Geometry check sheet. Reference: the model listing, model coordinates, mm. A direction names the side the tool comes from. Round coordinates to 2 decimals unless told otherwise and drop trailing zeros. Order: outer loops, then holes, each group sorted by start corner. A loop starts at its lowest first (then second) coordinate and runs counter-clockwise, first axis right, second up. Notation, with made-up numbers: (41, 32) - (80, 32) arc R20 cw to (80, 55) - close; hole circle Ø8 at (54, -21.5). An arc over 180 degrees is marked (long way). One line per question, with ' | ' between items. Start each with the question number.
Q1. Material ranges on line 1 along Y through (x, z) = (5, 25); line 2 along X through (y, z) = (15.5, 14.5); line 3 along Y through (x, z) = (38.1, 48.1), recorded low to high.
Q2. Tool access check on faces 1 (the face through (86.21, 34.72, 2.21)), 2 (the face through (107.95, 38, 26)), 3 (the face through (76.39, 41.44, 5.34)), 4 (the face through (13.99, 59.256, 47.669)), 5 (the face through (48, 0, 46)). Record the directions out of +Z, -Z, +X, -X, +Y, -Y that give a thin tool (end or side, any length) a straight path to the whole face; none if there is none.
Q3. Sectioned sample at D-D, the plane z = 12. Enter the section's corners in (x, y).
Q4. Sectioned sample at A-A, the plane y = 53. Enter the section's corners in (x, z).
Q5. Sectioned sample at C-C, the plane z = 25.4. Enter the section's corners in (x, y), then the cut area to 3 significant figures.
Q6. Sectioned sample at B-B, the plane x = 67. Enter the section's corners in (y, z), then the cut area to 3 significant figures.
Q7. Mould release check, pull along X, two halves, no side actions. Record for faces 6 (the face through (48, 76.2, 46)), 7 (the face through (0, 38, 26)), 8 (the face through (114.3, 38, 26)), 9 (the face through (109.934, 20.9, 21.6)): +X half, -X half, draft (parallel to the pull), parting line (faces both ways), or undercut.
```python
from build123d import *

# Parameters (mm, degrees)
SKETCH1_W           = 114.3
SKETCH1_H           = 50.8
SKETCH1_W_2         = 101.6
SKETCH1_H_2         = 38.1
BOSS_EXTRUDE1_DEPTH = 76.2
CUT_EXTRUDE1_REACH  = 148.464
SKETCH2_R           = 2.4765
SKETCH2_5_R         = 3.81
CUT_EXTRUDE2_DEPTH  = 147.463544952
SKETCH5_R           = 3.81
CUT_EXTRUDE4_DEPTH  = 147.463544952
SKETCH6_R           = 3.81
CUT_EXTRUDE5_DEPTH  = 147.463544952
SKETCH7_R           = 8.73125
CUT_EXTRUDE6_DEPTH  = 1.984375
SKETCH8_R           = 8.73125
CUT_EXTRUDE7_DEPTH  = 1.984375
CUT_EXTRUDE8_START  = -1.984375
SKETCH9_R           = 8.73125
CUT_EXTRUDE8_DEPTH  = 1.984375
CUT_EXTRUDE9_START  = -1.984375
SKETCH10_R          = 8.73125
CUT_EXTRUDE9_DEPTH  = 1.984375


with BuildPart() as part:
    # Sketch1 → Boss-Extrude1 (new body)
    with BuildSketch(Plane(origin=(0, 0, 0), x_dir=(1, 0, 0), z_dir=(0, 1, 0))):
        with Locations((57.15, -25.4)):
            Rectangle(SKETCH1_W, SKETCH1_H)
        with Locations((57.15, -25.4)):
            Rectangle(SKETCH1_W_2, SKETCH1_H_2, mode=Mode.SUBTRACT)
    extrude(amount=BOSS_EXTRUDE1_DEPTH)

    # Sketch2 → Cut-Extrude1 (cut, up to next)
    with BuildSketch(Plane.XY.offset(50.8), mode=Mode.PRIVATE) as cut_extrude1_sk1:
        with Locations((14.526827682, 61.673172318)):
            Circle(SKETCH2_R)
    cut_extrude1_tool1 = extrude(cut_extrude1_sk1.sketch, amount=-CUT_EXTRUDE1_REACH, mode=Mode.PRIVATE) & part.part
    # Sketch2 → Cut-Extrude1 (cut, up to next)
    with BuildSketch(Plane.XY.offset(50.8), mode=Mode.PRIVATE) as cut_extrude1_sk2:
        with Locations((61.673172318, 61.673172318)):
            Circle(SKETCH2_R)
    cut_extrude1_tool2 = extrude(cut_extrude1_sk2.sketch, amount=-CUT_EXTRUDE1_REACH, mode=Mode.PRIVATE) & part.part
    # Sketch2 → Cut-Extrude1 (cut, up to next)
    with BuildSketch(Plane.XY.offset(50.8), mode=Mode.PRIVATE) as cut_extrude1_sk3:
        with Locations((61.673172318, 14.526827682)):
            Circle(SKETCH2_R)
    cut_extrude1_tool3 = extrude(cut_extrude1_sk3.sketch, amount=-CUT_EXTRUDE1_REACH, mode=Mode.PRIVATE) & part.part
    # Sketch2 → Cut-Extrude1 (cut, up to next)
    with BuildSketch(Plane.XY.offset(50.8), mode=Mode.PRIVATE) as cut_extrude1_sk4:
        with Locations((14.526827682, 14.526827682)):
            Circle(SKETCH2_R)
    cut_extrude1_tool4 = extrude(cut_extrude1_sk4.sketch, amount=-CUT_EXTRUDE1_REACH, mode=Mode.PRIVATE) & part.part
    add(cut_extrude1_tool1.solids().sort_by_distance((14.526828, 61.673172, 50.8))[0], mode=Mode.SUBTRACT)
    add(cut_extrude1_tool2.solids().sort_by_distance((61.673172, 61.673172, 50.8))[0], mode=Mode.SUBTRACT)
    add(cut_extrude1_tool3.solids().sort_by_distance((61.673172, 14.526828, 50.8))[0], mode=Mode.SUBTRACT)
    add(cut_extrude1_tool4.solids().sort_by_distance((14.526828, 14.526828, 50.8))[0], mode=Mode.SUBTRACT)

    # Sketch2_5 → Cut-Extrude2 (cut, through all)
    with BuildSketch(Plane.XY.offset(50.8)):
        with Locations((38.1, 38.1)):
            Circle(SKETCH2_5_R)
    extrude(amount=-CUT_EXTRUDE2_DEPTH, mode=Mode.SUBTRACT)

    # Sketch5 → Cut-Extrude4 (cut, through all)
    with BuildSketch(Plane.XY.offset(50.8)):
        with Locations((84.455, 38.1)):
            Circle(SKETCH5_R)
    extrude(amount=-CUT_EXTRUDE4_DEPTH, mode=Mode.SUBTRACT)

    # Sketch6 → Cut-Extrude5 (cut, through all)
    with BuildSketch(Plane.ZY):
        with Locations((25.4, 19.05)):
            Circle(SKETCH6_R)
    extrude(amount=-CUT_EXTRUDE5_DEPTH, mode=Mode.SUBTRACT)

    # Sketch7 → Cut-Extrude6 (cut)
    with BuildSketch(Plane(origin=(6.35, 0, 0), x_dir=(0, 0, -1), z_dir=(1, 0, 0))):
        with Locations((-25.4, 19.05)):
            Circle(SKETCH7_R)
    extrude(amount=-CUT_EXTRUDE6_DEPTH, mode=Mode.SUBTRACT)

    # Sketch8 → Cut-Extrude7 (cut)
    with BuildSketch(Plane(origin=(0, 0, 44.45), x_dir=(-1, 0, 0), z_dir=(0, 0, -1))):
        with Locations((-38.1, 38.1)):
            Circle(SKETCH8_R)
        with Locations((-84.455, 38.1)):
            Circle(SKETCH8_R)
    extrude(amount=-CUT_EXTRUDE7_DEPTH, mode=Mode.SUBTRACT)

    # Sketch9 → Cut-Extrude8 (cut)
    with BuildSketch(Plane.ZY.offset(-107.95).offset(CUT_EXTRUDE8_START)):
        with Locations(Location((25.4, 19.05, 0), (0, 0, 180))):
            Circle(SKETCH9_R)
    extrude(amount=CUT_EXTRUDE8_DEPTH, mode=Mode.SUBTRACT)

    # Sketch10 → Cut-Extrude9 (cut)
    with BuildSketch(Plane.XY.offset(6.35).offset(CUT_EXTRUDE9_START)):
        with Locations(Location((38.1, 38.1, 0), (0, 0, 180))):
            Circle(SKETCH10_R)
        with Locations(Location((84.455, 38.1, 0), (0, 0, 180))):
            Circle(SKETCH10_R)
    extrude(amount=CUT_EXTRUDE9_DEPTH, mode=Mode.SUBTRACT)


solid = part.part
```
Determined:
1) line 1: y = 0 to 10.33, 27.77 to 76.2 | line 2: x = 0 to 6.35, 107.95 to 114.3 | line 3: y = 0 to 34.29, 41.91 to 76.2
2) face 1: +Z, -Z | face 2: +Y, -Y | face 3: none | face 4: +Z | face 5: +Z, -Z, +X, -X, -Y
3) outline: (0, 0) - (6.35, 0) - (6.35, 76.2) - (0, 76.2) - close; (107.95, 0) - (114.3, 0) - (114.3, 76.2) - (107.95, 76.2) - close
4) outline: (0, 0) - (114.3, 0) - (114.3, 50.8) - (0, 50.8) - close; hole (6.35, 6.35) - (107.95, 6.35) - (107.95, 44.45) - (6.35, 44.45) - close
5) outline: (0, 0) - (6.35, 0) - (6.35, 10.32) - (4.37, 10.32) - (4.37, 15.24) - (0, 15.24) - close; (0, 22.86) - (4.37, 22.86) - (4.37, 27.78) - (6.35, 27.78) - (6.35, 76.2) - (0, 76.2) - close; (107.95, 0) - (114.3, 0) - (114.3, 15.24) - (109.93, 15.24) - (109.93, 10.32) - (107.95, 10.32) - close; (107.95, 27.78) - (109.93, 27.78) - (109.93, 22.86) - (114.3, 22.86) - (114.3, 76.2) - (107.95, 76.2) - close | area: 832 mm2
6) outline: (0, 0) - (76.2, 0) - (76.2, 6.35) - (0, 6.35) - close; (0, 44.45) - (76.2, 44.45) - (76.2, 50.8) - (0, 50.8) - close | area: 968 mm2
7) face 6: draft | face 7: -X half | face 8: +X half | face 9: undercut
